```python
from build123d import *

# Parameters (mm, degrees)
SKETCH1_R           = 5.75
BOSS_EXTRUDE2_DEPTH = 3
BOSS_EXTRUDE3_DEPTH = 0.15
CIRPATTERN1_COUNT   = 2
SKETCH7_R           = 2.5
CUT_EXTRUDE1_DEPTH  = 65.252141201
FILLET1_R           = 1


with BuildPart() as part:
    # Sketch1 → Boss-Extrude2 (new, symmetric)
    with BuildSketch(Plane(origin=(0, 0, 0), x_dir=(1, 0, 0), z_dir=(0, 1, 0))):
        with Locations(Location((0, 0, 0), (0, 0, 270))):
            Circle(SKETCH1_R)
    extrude(amount=BOSS_EXTRUDE2_DEPTH, both=True)

    # Sketch6 → Boss-Extrude3 (add, symmetric)
    with BuildSketch(Plane(origin=(0, 0, 0), x_dir=(0.9743700647852352, -0.22495105434386534, 0), z_dir=(-0.2249510543438653, -0.9743700647852351, 0))):
        with BuildLine():
            Line((-5.557419516, 2.82), (-7.920891538, 5.18))
            Line((-7.920891538, 5.18), (-7.920891538, 63.5))
            Line((-7.920891538, 63.5), (-3.710891538, 63.5))
            ThreePointArc((-3.710891538, 63.5), (-0.694973133, 62.488011556), (1.100115443, 59.861694468))
            ThreePointArc((1.100115443, 59.861694468), (5.738056471, 28.958255312), (2.470780015, -2.12))
            ThreePointArc((2.470780015, -2.12), (-0.066255988, 2.750437774), (-5.557419516, 2.82))
        make_face()
    boss_extrude3 = extrude(amount=BOSS_EXTRUDE3_DEPTH, both=True)

    # CirPattern1: Boss-Extrude3 ×2 about axis
    cirpattern1_axis = Axis((0, 0, 0), (0, 1, 0))
    for i in range(1, CIRPATTERN1_COUNT):
        add(boss_extrude3.rotate(cirpattern1_axis, i * 360 / CIRPATTERN1_COUNT))

    # Sketch7 → Cut-Extrude1 (cut, through all)
    with BuildSketch(Plane(origin=(0, 3, 0), x_dir=(1, 0, 0), z_dir=(0, 1, 0))):
        with Locations(Location((0, 0, 0), (0, 0, 270))):
            Circle(SKETCH7_R)
    extrude(amount=-CUT_EXTRUDE1_DEPTH, mode=Mode.SUBTRACT)

    # Fillet1
    fillet1_edges = [part.edges().sort_by_distance(p)[0] for p in [
        (0, -3, -2.5),
        (0, 3, -2.5),
    ]]
    fillet(fillet1_edges, radius=FILLET1_R)


solid = part.part
```
For this review, take the finished solid that the model builds, in its own axes (mm). A direction names the side the tool comes from. Give positions to 0.01 mm unless a question says otherwise; leave off trailing zeros. Order: outer loops, then holes, each group sorted by start corner. A loop starts at its lowest first (then second) coordinate and runs counter-clockwise, first axis right, second up.
1) The part is to be moulded in two halves that separate along Z. For faces 3 (the face through (-2.44, 0.03, -0.54)), 4 (the face through (0.922, 0.367, -33.585)), say which applies: released by +Z, released by -Z, zero draft, split by the parting line, or undercut.
2) Take a section at B-B (z = -37.5). Give the boundary of the cut face in (x, y).
3) Insertion check: pin 1 (8 mm diameter, centred on x = -3.5, z = 17.5, fed in from -Y); pin 2 (6.5 mm diameter, centred on x = 0, z = 0, fed in from +Y); pin 3 (1 mm diameter, centred on x = 5, z = -13, fed in from +Y). Each pin has a flat end and moves straight along its axis. Give the tip position at first contact, or say it passes through.
4) For faces 1 (the face through (1.727, 0.042, 5.484)), 2 (the face through (0, -3, 4)), list the 3-axis set-ups (+Z, -Z, +X, -X, +Y, -Y) from which the entire face can be reached by the end or side of a thin tool; tool diameter is ignored.
5) Take a section at A-A (z = 0). Give the boundary of the cut face in (x, y), then the cut area to 3 significant figures.
6) Wall thickness on line 1 (X direction, y = -0.7, z = 0); line 2 (Z direction, x = -1.25, y = 1.75); line 3 (Z direction, x = -0.75, y = 1): over which ranges is each line inside the solid? List them lowest first.
Derived:
1. face 3: undercut
1. face 4: zero draft
2. outline: (-5.15, -1.04) - (-5.08, -1.33) - (7.75, 1.64) - (7.68, 1.93) - close
3. pin 1: stops at y = -0.27
3. pin 2: stops at y = 2.97
3. pin 3: stops at y = 1.42
4. face 1: none
4. face 2: +Z, -Z, +X, -X, -Y
5. outline: (-5.75, -3) - (-3.5, -3) arc R1 ccw to (-2.5, -2) - (-2.5, 2) arc R1 ccw to (-3.5, 3) - (-5.75, 3) - close; (2.5, -2) arc R1 ccw to (3.5, -3) - (5.75, -3) - (5.75, 3) - (3.5, 3) arc R1 ccw to (2.5, 2) - close
5. area: 38.1 mm2
6. line 1: x = -5.75 to -2.5, 2.5 to 5.75
6. line 2: z = -5.61 to -2.17, 2.17 to 5.61
6. line 3: z = -5.7 to -2.38, 2.38 to 5.7
